Autodesk Inventor part; units mm, degrees
ref_plane "YZ Plane" through (0, 0, 0) normal (1, 0, 0) x (0, 1, 0)
ref_plane "XZ Plane" through (0, 0, 0) normal (0, 1, 0) x (-1, 0, 0)
ref_plane "XY Plane" through (0, 0, 0) normal (0, 0, 1) x (1, 0, 0)
sketch "Boceto1" plane through (0, 0, 0) normal (0, 0, 1) x (1, 0, 0)
  arc A0 (-116.1173, -7.6512) -> (-117.6673, -9.2012) centre (-116.1173, -9.2012) ccw
  arc A1 (-117.6673, -9.2012) -> (-116.1173, -10.7512) centre (-116.1173, -9.2012) ccw
  arc A2 (-116.1173, -10.7512) -> (-114.5673, -9.2012) centre (-116.1173, -9.2012) ccw
  arc A3 (-114.5673, -9.2012) -> (-116.1173, -7.6512) centre (-116.1173, -9.2012) ccw
  arc A4 (-116.1173, -36.6512) -> (-117.6673, -38.2012) centre (-116.1173, -38.2012) ccw
  arc A5 (-117.6673, -38.2012) -> (-116.1173, -39.7512) centre (-116.1173, -38.2012) ccw
  arc A6 (-116.1173, -39.7512) -> (-114.5673, -38.2012) centre (-116.1173, -38.2012) ccw
  arc A7 (-114.5673, -38.2012) -> (-116.1173, -36.6512) centre (-116.1173, -38.2012) ccw
  arc A8 (-107.1173, -22.7512) -> (-112.0673, -27.7012) centre (-107.1173, -27.7012) ccw
  arc A9 (-112.0673, -27.7012) -> (-107.1173, -32.6512) centre (-107.1173, -27.7012) ccw
  arc A10 (-107.1173, -32.6512) -> (-102.1673, -27.7012) centre (-107.1173, -27.7012) ccw
  arc A11 (-102.1673, -27.7012) -> (-107.1173, -22.7512) centre (-107.1173, -27.7012) ccw
  line L0 (-98.1709, -2.0012) -> (-111.9173, -2.0012)
  line L1 (-111.9173, -2.0012) -> (-111.9173, 0.4988)
  line L2 (-111.9173, 0.4988) -> (-122.3173, 0.4988)
  line L3 (-122.3173, 0.4988) -> (-122.3173, -42.9012)
  line L4 (-122.3173, -42.9012) -> (-98.1709, -42.9012)
  line L5 (-98.1709, -42.9012) -> (-98.1709, -2.0012)
  point P0 (0, 0)
extrude "Extrusión1" add sketch "Boceto1" along normal blind 5
properties part number "carro x lado motor pieza 2 especial2"
Check sheet for the modelled part. Datum: model origin and axes. Units: mm. A direction names the side the tool comes from. Coordinates: 2 decimals unless noted, no trailing zeros. Write each loop counter-clockwise with the first axis right and the second up, starting at its lowest first coordinate (ties: lowest second). Pieces come first, ordered by that corner, then holes. Notation, with made-up numbers: (82, 76.5) -> (126, 76.5) arc R21 cw to (126, 85.5) -> close; hole circle Ø1 at (53.5, -24). An arc over 180 degrees is marked (long way). Use a Markdown table: item, result.
1. Sectioned sample at A-A (x = -106.5). Enter the section's corners in (y, z).
Reported:
| item | result |
|---|---|
| outline | (-42.9, 0) -> (-32.61, 0) -> (-32.61, 5) -> (-42.9, 5) -> close; (-22.79, 0) -> (-2, 0) -> (-2, 5) -> (-22.79, 5) -> close |
2. Sectioned sample at D-D (z = 3.4). Enter the section's corners in (x, y).
Reported:
| item | result |
|---|---|
| outline | (-122.32, -42.9) -> (-98.17, -42.9) -> (-98.17, -2) -> (-111.92, -2) -> (-111.92, 0.5) -> (-122.32, 0.5) -> close; hole circle Ø3.1 at (-116.12, -38.2); hole circle Ø3.1 at (-116.12, -9.2); hole circle Ø9.9 at (-107.12, -27.7) |
3. Tool access check on faces 1 (the flat face through (-110, -21, 5)), 2 (the flat face through (-105, -2.001, 2)). Record the directions out of +Z, -Z, +X, -X, +Y, -Y that give a thin tool (end or side, any length) a straight path to the whole face; none if there is none.
Reported:
| item | result |
|---|---|
| face 1 | +Z, +X, -X, +Y, -Y |
| face 2 | +Z, -Z, +X, +Y |
4. Go/stop test with flat-tipped pins: pin 1 Ø5 at (x, y) = (-116.12, -9.2) entering from +Z; pin 2 Ø1.2 at (y, z) = (-1, 2.5) entering from +X. Record where each tip stops, or that it passes through.
Reported:
| item | result |
|---|---|
| pin 1 | stops at z = 5 |
| pin 2 | stops at x = -111.92 |
5. Release check for a two-part mould opening along Y. For faces 3 (the cylindrical face through (-102.172, -27.484, 2.465)), 4 (the flat face through (-117, 0.499, 2)), 5 (the flat face through (-111.917, -1, 2)) record: pulls with the +Y half, pulls with the -Y half, needs draft (parallel to the pull), parting line crosses it, or undercut.
Reported:
| item | result |
|---|---|
| face 3 | undercut |
| face 4 | pulls with the +Y half |
| face 5 | needs draft |
6. Sectioned sample at C-C (x = -117). Enter the section's corners in (y, z), plus the area to 3 significant figures.
Reported:
| item | result |
|---|---|
| outline | (-42.9, 0) -> (-39.48, 0) -> (-39.48, 5) -> (-42.9, 5) -> close; (-36.93, 0) -> (-10.48, 0) -> (-10.48, 5) -> (-36.93, 5) -> close; (-7.93, 0) -> (0.5, 0) -> (0.5, 5) -> (-7.93, 5) -> close |
| area | 192 mm2 |
7. Sectioned sample at B-B (y = -32). Enter the section's corners in (x, z), plus the area to 3 significant figures.
Reported:
| item | result |
|---|---|
| outline | (-122.32, 0) -> (-109.57, 0) -> (-109.57, 5) -> (-122.32, 5) -> close; (-104.66, 0) -> (-98.17, 0) -> (-98.17, 5) -> (-104.66, 5) -> close |
| area | 96.2 mm2 |
8. Scan lines: line 1 along Y through (x, z) = (-116, 4.65); line 2 along Y through (x, z) = (-100.25, 0.7); line 3 along Y through (x, z) = (-117.25, 3.5). Record each from-to range of solid material in increasing order.
Reported:
| item | result |
|---|---|
| line 1 | y = -42.9 to -39.75, -36.66 to -10.75, -7.66 to 0.5 |
| line 2 | y = -42.9 to -2 |
| line 3 | y = -42.9 to -39.26, -37.14 to -10.26, -8.14 to 0.5 |
